Check sheet for the modelled part. Datum: model origin and axes. Units: mm. Round coordinates to 2 decimals unless told otherwise and drop trailing zeros. Write each loop counter-clockwise with the first axis right and the second up, starting at its lowest first coordinate (ties: lowest second). Pieces come first, ordered by that corner, then holes. Notation, with made-up numbers: M -21,-6.75 L -13,-6.75 A8 cw -13,6.25 Z; hole C 70,2 d3. An arc over 180 degrees is marked long. One line per item, written item: value.
from build123d import *

# Parameters (mm, degrees)
F2_W     = 24
F2_H     = 90
F2_R     = 6.75
F3_DEPTH = 5
F4_R     = 10
F5_W     = 5
F5_H     = 5
F6_DEPTH = 25
F7_R     = 1


with BuildPart() as f3:
    # F2 (on Front) → F3 (new body)
    with BuildSketch(Plane.XZ):
        with Locations((12, 45)):
            Rectangle(F2_W, F2_H)
        with Locations((12, 12)):
            Circle(F2_R, mode=Mode.SUBTRACT)
        with Locations((12, 60)):
            Circle(F2_R, mode=Mode.SUBTRACT)
    extrude(amount=F3_DEPTH)

    # F4
    f4_edges = [f3.edges().sort_by_distance(p)[0] for p in [
        (0, -2.5, 90),
        (0, -2.5, 0),
        (24, -2.5, 90),
        (24, -2.5, 0),
    ]]
    fillet(f4_edges, radius=F4_R)

    # F5 (on face) → F6 (cut)
    with BuildSketch(Plane.XZ.offset(5)):
        with BuildLine():
            Line((19, 81), (19, 76))
            Line((19, 76), (24, 76))
            Line((24, 76), (24, 80))
            ThreePointArc((24, 80), (23.9874607311, 80.5006277506), (23.9498743711, 81))
            Line((23.9498743711, 81), (19, 81))
        make_face()
        with Locations((21.5, 43.25)):
            Rectangle(F5_W, F5_H)
        with Locations((21.5, 28.75)):
            Rectangle(F5_W, F5_H)
    extrude(amount=-F6_DEPTH, mode=Mode.SUBTRACT)

    # F7
    f7_edges = [f3.edges().sort_by_distance(p)[0] for p in [
        (24, -2.5, 26.25),
        (24, -2.5, 31.25),
        (24, -2.5, 40.75),
        (24, -2.5, 45.75),
        (24, -2.5, 76),
        (23.949874, -2.5, 81),
    ]]
    fillet(f7_edges, radius=F7_R)


solid = f3.part
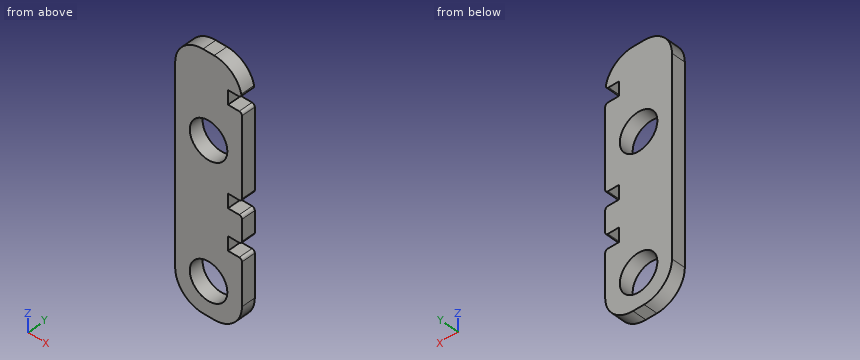
Q1. Depth check by flat-ended pin: P1, Ø1, axis at x = 4.5, z = 17, coming from the +Y side; P2, Ø1, axis at x = 21, y = -2, coming from the -Z side; P3, Ø3, axis at x = 21.5, y = -2, coming from the -Z side; P4, Ø1.2, axis at x = 20.5, y = -2, coming from the +Z side. Enter the tip coordinate at first touch or a pass-through.
Completed:
P1: y = 0
P2: z = 2.4
P3: z = 2
P4: z = 88.07
Q2. Sectioned sample at D-D on x = 7. Enter the section's corners in (y, z), and give its area (3 significant figures).
Completed:
outline: M -5,0.46 L 0,0.46 L 0,7.47 L -5,7.47 Z; M -5,16.53 L 0,16.53 L 0,55.47 L -5,55.47 Z; M -5,64.53 L 0,64.53 L 0,89.54 L -5,89.54 Z
area: 355 mm^2
Q3. Sectioned sample at A-A on z = 60. Enter the section's corners in (x, y).
Completed:
outline: M 0,-5 L 5.25,-5 L 5.25,0 L 0,0 Z; M 18.75,-5 L 24,-5 L 24,0 L 18.75,0 Z
Q4. Scan lines: line 1 (Z direction, x = 12, y = -2.9); line 2 (Z direction, x = 6.5, y = -2.35); line 3 (Z direction, x = 20, y = -1.7). Record each from-to range of solid material in increasing order. Write a range as [from, to].
Completed:
line 1: [0, 5.25], [18.75, 53.25], [66.75, 90]
line 2: [0.63, 8.09], [15.91, 56.09], [63.91, 89.37]
line 3: [2, 26.25], [31.25, 40.75], [45.75, 76], [81, 88]
Q5. Sectioned sample at B-B on x = 12. Enter the section's corners in (y, z).
Completed:
outline: M -5,0 L 0,0 L 0,5.25 L -5,5.25 Z; M -5,18.75 L 0,18.75 L 0,53.25 L -5,53.25 Z; M -5,66.75 L 0,66.75 L 0,90 L -5,90 Z
Q6. Sectioned sample at C-C on y = -2.3. Enter the section's corners in (x, z), and give its area (3 significant figures).
Completed:
outline: M 0,10 A10 ccw 10,0 L 14,0 A10 ccw 24,10 L 24,25.25 A1 ccw 23,26.25 L 19,26.25 L 19,31.25 L 23,31.25 A1 ccw 24,32.25 L 24,39.75 A1 ccw 23,40.75 L 19,40.75 L 19,45.75 L 23,45.75 A1 ccw 24,46.75 L 24,75 A1 ccw 23,76 L 19,76 L 19,81 L 22.77,81 A1 ccw 23.75,82.22 A10 ccw 14,90 L 10,90 A10 ccw 0,80 Z; hole C 12,12 d13.5; hole C 12,60 d13.5
area: 1,710 mm^2
